from build123d import *

# Parameters (mm, degrees)
MODEL_R                 = 1.5
MODEL_R_2               = 6
SALIENTE_EXTRUIR1_DEPTH = 3


with BuildPart() as part:
    # Model → Saliente-Extruir1 (new body)
    with BuildSketch(Plane.XY):
        with BuildLine():
            Line((187.952926253, 215.611282897), (189.952926253, 215.611282897))
            Line((189.952926253, 215.611282897), (189.952926253, 224.611282897))
            Line((189.952926253, 224.611282897), (212.452926253, 224.611282897))
            Line((212.452926253, 224.611282897), (212.452926253, 197.611282897))
            Line((212.452926253, 197.611282897), (207.952926253, 197.611282897))
            Line((207.952926253, 197.611282897), (207.952926253, 195.611282897))
            Line((207.952926253, 195.611282897), (197.952926253, 195.611282897))
            Line((197.952926253, 195.611282897), (197.952926253, 190.611282897))
            Line((197.952926253, 190.611282897), (207.952926253, 190.611282897))
            Line((207.952926253, 190.611282897), (207.952926253, 188.611282897))
            Line((207.952926253, 188.611282897), (212.452926253, 188.611282897))
            Line((212.452926253, 188.611282897), (212.452926253, 183.995647927))
            Line((212.452926253, 183.995647927), (205.452926253, 178.111282897))
            ThreePointArc((205.452926253, 178.111282897), (203.988460159, 174.575748991), (200.452926253, 173.111282897))
            Line((200.452926253, 173.111282897), (170.452926253, 173.111282897))
            ThreePointArc((170.452926253, 173.111282897), (166.917392347, 174.575748991), (165.452926253, 178.111282897))
            Line((165.452926253, 178.111282897), (158.452926253, 183.995647927))
            Line((158.452926253, 183.995647927), (158.452926253, 188.611282897))
            Line((158.452926253, 188.611282897), (162.952926253, 188.611282897))
            Line((162.952926253, 188.611282897), (162.952926253, 190.611282897))
            Line((162.952926253, 190.611282897), (172.952926253, 190.611282897))
            Line((172.952926253, 190.611282897), (172.952926253, 195.611282897))
            Line((172.952926253, 195.611282897), (162.952926253, 195.611282897))
            Line((162.952926253, 195.611282897), (162.952926253, 197.611282897))
            Line((162.952926253, 197.611282897), (158.452926253, 197.611282897))
            Line((158.452926253, 197.611282897), (158.452926253, 224.611282897))
            Line((158.452926253, 224.611282897), (180.952926253, 224.611282897))
            Line((180.952926253, 224.611282897), (180.952926253, 215.611282897))
            Line((180.952926253, 215.611282897), (182.952926253, 215.611282897))
            Line((182.952926253, 215.611282897), (182.952926253, 205.611282897))
            Line((182.952926253, 205.611282897), (187.952926253, 205.611282897))
            Line((187.952926253, 205.611282897), (187.952926253, 215.611282897))
        make_face()
        with Locations((207.952926253, 220.111282897)):
            Circle(MODEL_R, mode=Mode.SUBTRACT)
        with Locations((200.452926253, 208.111282897)):
            Circle(MODEL_R, mode=Mode.SUBTRACT)
        with Locations((207.952926253, 184.111282897)):
            Circle(MODEL_R, mode=Mode.SUBTRACT)
        with Locations((185.452926253, 193.111282897)):
            Circle(MODEL_R_2, mode=Mode.SUBTRACT)
        with Locations((200.452926253, 178.111282897)):
            Circle(MODEL_R, mode=Mode.SUBTRACT)
        with Locations((162.952926253, 220.111282897)):
            Circle(MODEL_R, mode=Mode.SUBTRACT)
        with Locations((170.452926253, 208.111282897)):
            Circle(MODEL_R, mode=Mode.SUBTRACT)
        with Locations((162.952926253, 184.111282897)):
            Circle(MODEL_R, mode=Mode.SUBTRACT)
        with Locations((170.452926253, 178.111282897)):
            Circle(MODEL_R, mode=Mode.SUBTRACT)
        with BuildLine():
            Line((169.702926253, 221.611282897), (174.202926253, 221.611282897))
            ThreePointArc((174.202926253, 221.611282897), (175.702926253, 220.111282897), (174.202926253, 218.611282897))
            Line((174.202926253, 218.611282897), (169.702926253, 218.611282897))
            ThreePointArc((169.702926253, 218.611282897), (168.202926253, 220.111282897), (169.702926253, 221.611282897))
        make_face(mode=Mode.SUBTRACT)
        with BuildLine():
            Line((164.452926253, 208.861282897), (164.452926253, 204.361282897))
            ThreePointArc((164.452926253, 204.361282897), (162.952926253, 202.861282897), (161.452926253, 204.361282897))
            Line((161.452926253, 204.361282897), (161.452926253, 208.861282897))
            ThreePointArc((161.452926253, 208.861282897), (162.952926253, 210.361282897), (164.452926253, 208.861282897))
        make_face(mode=Mode.SUBTRACT)
        with BuildLine():
            Line((196.702926253, 218.611282897), (201.202926253, 218.611282897))
            ThreePointArc((201.202926253, 218.611282897), (202.702926253, 220.111282897), (201.202926253, 221.611282897))
            Line((201.202926253, 221.611282897), (196.702926253, 221.611282897))
            ThreePointArc((196.702926253, 221.611282897), (195.202926253, 220.111282897), (196.702926253, 218.611282897))
        make_face(mode=Mode.SUBTRACT)
        with BuildLine():
            Line((206.452926253, 208.861282897), (206.452926253, 204.361282897))
            ThreePointArc((206.452926253, 204.361282897), (207.952926253, 202.861282897), (209.452926253, 204.361282897))
            Line((209.452926253, 204.361282897), (209.452926253, 208.861282897))
            ThreePointArc((209.452926253, 208.861282897), (207.952926253, 210.361282897), (206.452926253, 208.861282897))
        make_face(mode=Mode.SUBTRACT)
    extrude(amount=SALIENTE_EXTRUIR1_DEPTH)


solid = part.part
Work out the finished part from the listing and answer in its coordinate system (mm). A direction names the side the tool comes from. Give positions to 0.01 mm unless a question says otherwise; leave off trailing zeros. Order: outer loops, then holes, each group sorted by start corner. A loop starts at its lowest first (then second) coordinate and runs counter-clockwise, first axis right, second up. Notation, with made-up numbers: (2, 40.25) - (8, 40.25) arc R8 cw to (8, 55.25) - close; hole circle Ø10 at (48, -17). An arc over 180 degrees is marked (long way). Answer as CSV lines item,"result". Start each with the question number.
Q1. Find the intervals of material crossed by L1, parallel to X at y = 208, z = 1.45; L2, parallel to X at y = 213, z = 2.3; L3, parallel to X at y = 216.5, z = 2.6, in increasing order. Write a range as [from, to].
Q2. The part is cut by section A-A (y = 213). Write down the section's boundary in (x, z).
Q3. The part is cut by section C-C (z = 2.4). Give the number of separate pieces and of enclosed holes in the cut face, then the cut area to 3 significant figures.
Q4. Given pin 1 Ø1.5 at (y, z) = (194, 2) entering from +X; pin 2 Ø0.6 at (y, z) = (189.5, 1.5) entering from +X; pin 3 Ø0.6 at (x, z) = (189.5, 1) entering from +Y, each flat-ended and moving along its own axis, determine where each tip first touches the part or whether it passes through.
Q5. The part is cut by section B-B (x = 182). Write down the section's boundary in (y, z), then the cut area to 3 significant figures.
Q6. The part is cut by section D-D (y = 181.5). Write down the section's boundary in (x, z).
Q7. The mould has two halves that part along Y. Classify faces 4 (the face through (204.027, 174.615, 1.479)), 5 (the face through (187.953, 211, 1)), 6 (the face through (207.99, 210.36, 1.48)), 7 (the face through (185, 205.611, 1)): +Y half, -Y half, draft (parallel to the pull), parting line (faces both ways), or undercut.
Q8. For faces 1 (the face through (203, 190.611, 1)), 2 (the face through (168.203, 220.078, 1.479)), 3 (the face through (161, 188.611, 1)), determine the directions among +Z, -Z, +X, -X, +Y, -Y from which every point of the face is accessible in a straight line to the end or side of a thin tool.
Check result:
1,L1,"x = [158.45, 161.45], [164.45, 168.96], [171.95, 182.95], [187.95, 198.96], [201.95, 206.45], [209.45, 212.45]"
1,L2,"x = [158.45, 182.95], [187.95, 212.45]"
1,L3,"x = [158.45, 180.95], [189.95, 212.45]"
2,outline,"(158.45, 0) - (182.95, 0) - (182.95, 3) - (158.45, 3) - close; (187.95, 0) - (212.45, 0) - (212.45, 3) - (187.95, 3) - close"
3,separate pieces,"1"
3,enclosed holes,"13"
3,area,"2,100 mm²"
4,pin 1,"stops at x = 197.95"
4,pin 2,"stops at x = 207.95"
4,pin 3,"stops at y = 215.61"
5,outline,"(173.11, 0) - (188.2, 0) - (188.2, 3) - (173.11, 3) - close; (198.02, 0) - (215.61, 0) - (215.61, 3) - (198.02, 3) - close"
5,area,"98.1 mm²"
6,outline,"(161.42, 0) - (209.48, 0) - (209.48, 3) - (161.42, 3) - close"
7,face 4,"-Y half"
7,face 5,"draft"
7,face 6,"undercut"
7,face 7,"+Y half"
8,face 1,"+Z, -Z, +X"
8,face 2,"+Z, -Z"
8,face 3,"+Z, -Z, -X"
